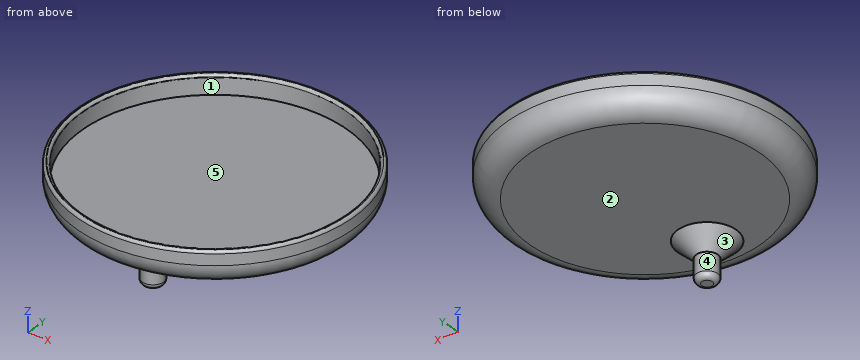
from build123d import *

# Parameters (mm, degrees)
BOSS_EXTRUDE1_DEPTH      = 3.75
BOSS_EXTRUDE1_DEPTH_BACK = 3.5
SKETCH1_R                = 1.95
SKETCH2_R                = 25
BOSS_EXTRUDE2_DEPTH      = 3
SKETCH3_R                = 25
SKETCH3_R_2              = 24
BOSS_EXTRUDE3_DEPTH      = 3.5
FILLET1_R                = 0.5
FILLET2_R                = 4
CHAMFER1_SIZE            = 3
CHAMFER1_SIZE2           = 3.331837544
FILLET3_R                = 1


with BuildPart() as part:
    # Sketch1 → Boss-Extrude1 (new, two sides: drawn at the far end of the back side and taken through both)
    with BuildSketch(Plane.XY.offset(-BOSS_EXTRUDE1_DEPTH_BACK)):
        Circle(SKETCH1_R)
    extrude(amount=BOSS_EXTRUDE1_DEPTH + BOSS_EXTRUDE1_DEPTH_BACK)

    # Sketch2 → Boss-Extrude2 (add)
    with BuildSketch(Plane.XY.offset(3.75)):
        with Locations((0, 14.750067334)):
            Circle(SKETCH2_R)
    extrude(amount=BOSS_EXTRUDE2_DEPTH)

    # Sketch3 → Boss-Extrude3 (add)
    with BuildSketch(Plane.XY.offset(6.75)):
        with Locations((0, 14.750067334)):
            Circle(SKETCH3_R)
        with Locations((0, 14.750067334)):
            Circle(SKETCH3_R_2, mode=Mode.SUBTRACT)
    extrude(amount=BOSS_EXTRUDE3_DEPTH)

    # Fillet1
    fillet1_edges = [part.edges().sort_by_distance(p)[0] for p in [
        (-25, 14.750067334, 10.25),
        (-24, 14.750067334, 10.25),
    ]]
    fillet(fillet1_edges, radius=FILLET1_R - 0.0001)  # a hair under: the kernel refuses the full size

    # Fillet2
    fillet2_edges = [part.edges().sort_by_distance(p)[0] for p in [
        (-25, 14.750067334, 3.75),
    ]]
    fillet(fillet2_edges, radius=FILLET2_R)

    # Chamfer1
    chamfer1_edges = [part.edges().sort_by_distance(p)[0] for p in [
        (-1.95, 0, 3.75),
    ]]
    chamfer1_side = [part.faces().sort_by_distance(p)[0] for p in [
        (-1.95, 0, 1.875),
    ]]
    chamfer(chamfer1_edges, length=CHAMFER1_SIZE, length2=CHAMFER1_SIZE2, reference=chamfer1_side[0])

    # Fillet3
    fillet3_edges = [part.edges().sort_by_distance(p)[0] for p in [
        (-1.95, 0, -3.5),
    ]]
    fillet(fillet3_edges, radius=FILLET3_R)


solid = part.part
Can you work these out from the model? Positions are in its coordinate system, mm. Face numbers are marked on the shaded views. A direction names the side the tool comes from. Round coordinates to 2 decimals unless told otherwise and drop trailing zeros. Write each loop counter-clockwise with the first axis right and the second up, starting at its lowest first coordinate (ties: lowest second). Pieces come first, ordered by that corner, then holes. Notation, with made-up numbers: M -5.75,76 L 20.25,76 A20 ccw 20.25,88 Z; hole C 34.25,86.25 d5. An arc over 180 degrees is marked long. Use a Markdown table: item, result.
Item 1: For pin 1 Ø24 at (x, y) = (7.5, 14.5) entering from +Z; pin 2 Ø3 at (y, z) = (31, 1) entering from -X; pin 3 Ø5 at (x, y) = (-18.5, 34) entering from -Z; pin 4 Ø10 at (x, y) = (17, 30.5) entering from +Z, each with a flat end and sliding along its axis, tell me the tip position at first contact or that it passes through.
Found:
| item | result |
|---|---|
| pin 1 | stops at z = 6.75 |
| pin 2 | passes through |
| pin 3 | stops at z = 5.35 |
| pin 4 | stops at z = 10.25 |
Item 2: Which directions (+Z, -Z, +X, -X, +Y, -Y) give clear straight access to the entire face, cutting with the end or side of a thin tool? Please do the marked faces 4 and 5.
Found:
| item | result |
|---|---|
| face 4 | -Z |
| face 5 | +Z |
Item 3: If I drill on line 1 along Y through (x, z) = (0, 8.4); line 2 along X through (y, z) = (11, 9); line 3 along Z through (x, y) = (-8.5, 21), over which ranges is the centre line in solid material (lowest first)? Write a range as [from, to].
Found:
| item | result |
|---|---|
| line 1 | y = [-10.25, -9.25], [38.75, 39.75] |
| line 2 | x = [-24.72, -23.71], [23.71, 24.72] |
| line 3 | z = [3.75, 6.75] |
Item 4: We'd pull the mould along Y, two halves only. Please class the marked faces 1, 2 and 3: released by +Y, released by -Y, zero draft, split by the parting line, or undercut.
Found:
| item | result |
|---|---|
| face 1 | undercut |
| face 2 | zero draft |
| face 3 | split by the parting line |
Item 5: I want a section at C-C (z = 5.5). List the corners of the cut face in (x, y) for me, and give its area (3 significant figures).
Found:
| item | result |
|---|---|
| outline | C 0,14.75 d48.61 |
| area | 1,860 mm2 |
Item 6: I want a section at B-B (z = 2.25). List the corners of the cut face in (x, y) for me.
Found:
| item | result |
|---|---|
| outline | C 0,0 d7.23 |
Item 7: I want a section at A-A (z = 8.5). List the corners of the cut face in (x, y) for me, and give its area (3 significant figures).
Found:
| item | result |
|---|---|
| outline | C 0,14.75 d50; hole C 0,14.75 d48 |
| area | 154 mm2 |
